Read the model definition and answer for the solid it produces. Units are mm, in the model's axes. A direction names the side the tool comes from. Give positions to 0.01 mm unless a question says otherwise; leave off trailing zeros. Order: outer loops, then holes, each group sorted by start corner. A loop starts at its lowest first (then second) coordinate and runs counter-clockwise, first axis right, second up. Notation, with made-up numbers: M 75.5,42.25 L 100.5,42.25 A22 ccw 100.5,55.25 Z; hole C 63.25,75 d8. An arc over 180 degrees is marked long. Write item = value, one per line. Start each with the question number.
from build123d import *

# Parameters (mm, degrees)
BOSS_EXTRUDE1_DEPTH = 1168.4
CUT_EXTRUDE1_REACH  = 27.4
SKETCH2_R           = 2.667
CUT_EXTRUDE2_REACH  = 27.4
SKETCH3_R           = 2.5527


with BuildPart() as part:
    # Sketch1 → Boss-Extrude1 (new body)
    with BuildSketch(Plane(origin=(0, 0, 0), x_dir=(1, 0, 0), z_dir=(0, 1, 0))):
        Polygon((3.175, 3.175), (3.175, 25.4), (0, 25.4), (0, 0), (50.8, 0), (50.8, 25.4), (47.625, 25.4), (47.625, 3.175), align=None)
    extrude(amount=BOSS_EXTRUDE1_DEPTH)

    # Sketch2 → Cut-Extrude1 (cut, up to next)
    with BuildSketch(Plane.XY, mode=Mode.PRIVATE) as cut_extrude1_sk1:
        with Locations((25.4, 76.2)):
            Circle(SKETCH2_R)
    cut_extrude1_tool1 = extrude(cut_extrude1_sk1.sketch, amount=-CUT_EXTRUDE1_REACH, mode=Mode.PRIVATE) & part.part
    add(cut_extrude1_tool1.solids().sort_by_distance((25.4, 76.2, 0))[0], mode=Mode.SUBTRACT)
    # Sketch2 → Cut-Extrude1 (cut, up to next)
    with BuildSketch(Plane.XY, mode=Mode.PRIVATE) as cut_extrude1_sk2:
        with Locations((25.4, 136.144)):
            Circle(SKETCH2_R)
    cut_extrude1_tool2 = extrude(cut_extrude1_sk2.sketch, amount=-CUT_EXTRUDE1_REACH, mode=Mode.PRIVATE) & part.part
    add(cut_extrude1_tool2.solids().sort_by_distance((25.4, 136.144, 0))[0], mode=Mode.SUBTRACT)
    # Sketch2 → Cut-Extrude1 (cut, up to next)
    with BuildSketch(Plane.XY, mode=Mode.PRIVATE) as cut_extrude1_sk3:
        with Locations((25.4, 196.088)):
            Circle(SKETCH2_R)
    cut_extrude1_tool3 = extrude(cut_extrude1_sk3.sketch, amount=-CUT_EXTRUDE1_REACH, mode=Mode.PRIVATE) & part.part
    add(cut_extrude1_tool3.solids().sort_by_distance((25.4, 196.088, 0))[0], mode=Mode.SUBTRACT)
    # Sketch2 → Cut-Extrude1 (cut, up to next)
    with BuildSketch(Plane.XY, mode=Mode.PRIVATE) as cut_extrude1_sk4:
        with Locations((25.4, 256.032)):
            Circle(SKETCH2_R)
    cut_extrude1_tool4 = extrude(cut_extrude1_sk4.sketch, amount=-CUT_EXTRUDE1_REACH, mode=Mode.PRIVATE) & part.part
    add(cut_extrude1_tool4.solids().sort_by_distance((25.4, 256.032, 0))[0], mode=Mode.SUBTRACT)
    # Sketch2 → Cut-Extrude1 (cut, up to next)
    with BuildSketch(Plane.XY, mode=Mode.PRIVATE) as cut_extrude1_sk5:
        with Locations((25.4, 315.976)):
            Circle(SKETCH2_R)
    cut_extrude1_tool5 = extrude(cut_extrude1_sk5.sketch, amount=-CUT_EXTRUDE1_REACH, mode=Mode.PRIVATE) & part.part
    add(cut_extrude1_tool5.solids().sort_by_distance((25.4, 315.976, 0))[0], mode=Mode.SUBTRACT)
    # Sketch2 → Cut-Extrude1 (cut, up to next)
    with BuildSketch(Plane.XY, mode=Mode.PRIVATE) as cut_extrude1_sk6:
        with Locations((25.4, 375.92)):
            Circle(SKETCH2_R)
    cut_extrude1_tool6 = extrude(cut_extrude1_sk6.sketch, amount=-CUT_EXTRUDE1_REACH, mode=Mode.PRIVATE) & part.part
    add(cut_extrude1_tool6.solids().sort_by_distance((25.4, 375.92, 0))[0], mode=Mode.SUBTRACT)
    # Sketch2 → Cut-Extrude1 (cut, up to next)
    with BuildSketch(Plane.XY, mode=Mode.PRIVATE) as cut_extrude1_sk7:
        with Locations((25.4, 435.864)):
            Circle(SKETCH2_R)
    cut_extrude1_tool7 = extrude(cut_extrude1_sk7.sketch, amount=-CUT_EXTRUDE1_REACH, mode=Mode.PRIVATE) & part.part
    add(cut_extrude1_tool7.solids().sort_by_distance((25.4, 435.864, 0))[0], mode=Mode.SUBTRACT)
    # Sketch2 → Cut-Extrude1 (cut, up to next)
    with BuildSketch(Plane.XY, mode=Mode.PRIVATE) as cut_extrude1_sk8:
        with Locations((25.4, 495.808)):
            Circle(SKETCH2_R)
    cut_extrude1_tool8 = extrude(cut_extrude1_sk8.sketch, amount=-CUT_EXTRUDE1_REACH, mode=Mode.PRIVATE) & part.part
    add(cut_extrude1_tool8.solids().sort_by_distance((25.4, 495.808, 0))[0], mode=Mode.SUBTRACT)
    # Sketch2 → Cut-Extrude1 (cut, up to next)
    with BuildSketch(Plane.XY, mode=Mode.PRIVATE) as cut_extrude1_sk9:
        with Locations((25.4, 555.752)):
            Circle(SKETCH2_R)
    cut_extrude1_tool9 = extrude(cut_extrude1_sk9.sketch, amount=-CUT_EXTRUDE1_REACH, mode=Mode.PRIVATE) & part.part
    add(cut_extrude1_tool9.solids().sort_by_distance((25.4, 555.752, 0))[0], mode=Mode.SUBTRACT)
    # Sketch2 → Cut-Extrude1 (cut, up to next)
    with BuildSketch(Plane.XY, mode=Mode.PRIVATE) as cut_extrude1_sk10:
        with Locations((25.4, 615.696)):
            Circle(SKETCH2_R)
    cut_extrude1_tool10 = extrude(cut_extrude1_sk10.sketch, amount=-CUT_EXTRUDE1_REACH, mode=Mode.PRIVATE) & part.part
    add(cut_extrude1_tool10.solids().sort_by_distance((25.4, 615.696, 0))[0], mode=Mode.SUBTRACT)
    # Sketch2 → Cut-Extrude1 (cut, up to next)
    with BuildSketch(Plane.XY, mode=Mode.PRIVATE) as cut_extrude1_sk11:
        with Locations((25.4, 675.64)):
            Circle(SKETCH2_R)
    cut_extrude1_tool11 = extrude(cut_extrude1_sk11.sketch, amount=-CUT_EXTRUDE1_REACH, mode=Mode.PRIVATE) & part.part
    add(cut_extrude1_tool11.solids().sort_by_distance((25.4, 675.64, 0))[0], mode=Mode.SUBTRACT)
    # Sketch2 → Cut-Extrude1 (cut, up to next)
    with BuildSketch(Plane.XY, mode=Mode.PRIVATE) as cut_extrude1_sk12:
        with Locations((25.4, 735.584)):
            Circle(SKETCH2_R)
    cut_extrude1_tool12 = extrude(cut_extrude1_sk12.sketch, amount=-CUT_EXTRUDE1_REACH, mode=Mode.PRIVATE) & part.part
    add(cut_extrude1_tool12.solids().sort_by_distance((25.4, 735.584, 0))[0], mode=Mode.SUBTRACT)
    # Sketch2 → Cut-Extrude1 (cut, up to next)
    with BuildSketch(Plane.XY, mode=Mode.PRIVATE) as cut_extrude1_sk13:
        with Locations((25.4, 795.528)):
            Circle(SKETCH2_R)
    cut_extrude1_tool13 = extrude(cut_extrude1_sk13.sketch, amount=-CUT_EXTRUDE1_REACH, mode=Mode.PRIVATE) & part.part
    add(cut_extrude1_tool13.solids().sort_by_distance((25.4, 795.528, 0))[0], mode=Mode.SUBTRACT)
    # Sketch2 → Cut-Extrude1 (cut, up to next)
    with BuildSketch(Plane.XY, mode=Mode.PRIVATE) as cut_extrude1_sk14:
        with Locations((25.4, 855.472)):
            Circle(SKETCH2_R)
    cut_extrude1_tool14 = extrude(cut_extrude1_sk14.sketch, amount=-CUT_EXTRUDE1_REACH, mode=Mode.PRIVATE) & part.part
    add(cut_extrude1_tool14.solids().sort_by_distance((25.4, 855.472, 0))[0], mode=Mode.SUBTRACT)
    # Sketch2 → Cut-Extrude1 (cut, up to next)
    with BuildSketch(Plane.XY, mode=Mode.PRIVATE) as cut_extrude1_sk15:
        with Locations((25.4, 915.416)):
            Circle(SKETCH2_R)
    cut_extrude1_tool15 = extrude(cut_extrude1_sk15.sketch, amount=-CUT_EXTRUDE1_REACH, mode=Mode.PRIVATE) & part.part
    add(cut_extrude1_tool15.solids().sort_by_distance((25.4, 915.416, 0))[0], mode=Mode.SUBTRACT)
    # Sketch2 → Cut-Extrude1 (cut, up to next)
    with BuildSketch(Plane.XY, mode=Mode.PRIVATE) as cut_extrude1_sk16:
        with Locations((25.4, 975.36)):
            Circle(SKETCH2_R)
    cut_extrude1_tool16 = extrude(cut_extrude1_sk16.sketch, amount=-CUT_EXTRUDE1_REACH, mode=Mode.PRIVATE) & part.part
    add(cut_extrude1_tool16.solids().sort_by_distance((25.4, 975.36, 0))[0], mode=Mode.SUBTRACT)
    # Sketch2 → Cut-Extrude1 (cut, up to next)
    with BuildSketch(Plane.XY, mode=Mode.PRIVATE) as cut_extrude1_sk17:
        with Locations((25.4, 1035.304)):
            Circle(SKETCH2_R)
    cut_extrude1_tool17 = extrude(cut_extrude1_sk17.sketch, amount=-CUT_EXTRUDE1_REACH, mode=Mode.PRIVATE) & part.part
    add(cut_extrude1_tool17.solids().sort_by_distance((25.4, 1035.304, 0))[0], mode=Mode.SUBTRACT)
    # Sketch2 → Cut-Extrude1 (cut, up to next)
    with BuildSketch(Plane.XY, mode=Mode.PRIVATE) as cut_extrude1_sk18:
        with Locations((25.4, 1095.248)):
            Circle(SKETCH2_R)
    cut_extrude1_tool18 = extrude(cut_extrude1_sk18.sketch, amount=-CUT_EXTRUDE1_REACH, mode=Mode.PRIVATE) & part.part
    add(cut_extrude1_tool18.solids().sort_by_distance((25.4, 1095.248, 0))[0], mode=Mode.SUBTRACT)

    # Sketch3 → Cut-Extrude2 (cut, up to next)
    with BuildSketch(Plane.XY, mode=Mode.PRIVATE) as cut_extrude2_sk1:
        with Locations((25.4, 32.131)):
            Circle(SKETCH3_R)
    cut_extrude2_tool1 = extrude(cut_extrude2_sk1.sketch, amount=-CUT_EXTRUDE2_REACH, mode=Mode.PRIVATE) & part.part
    add(cut_extrude2_tool1.solids().sort_by_distance((25.4, 32.131, 0))[0], mode=Mode.SUBTRACT)
    # Sketch3 → Cut-Extrude2 (cut, up to next)
    with BuildSketch(Plane.XY, mode=Mode.PRIVATE) as cut_extrude2_sk2:
        with Locations((25.4, 14.2875)):
            Circle(SKETCH3_R)
    cut_extrude2_tool2 = extrude(cut_extrude2_sk2.sketch, amount=-CUT_EXTRUDE2_REACH, mode=Mode.PRIVATE) & part.part
    add(cut_extrude2_tool2.solids().sort_by_distance((25.4, 14.2875, 0))[0], mode=Mode.SUBTRACT)


solid = part.part
1) Find the intervals of material crossed by probe 1 along X at (y, z) = (1019, -17.5) (3 decimals); probe 2 along Z at (x, y) = (19.5, 279.5) (3 decimals), in increasing order. Write a range as [from, to].
2) Find section A-A on z = -13. Determine the outline of the cut face in (x, y) (3 decimals).
3) For faces 1 (the face through (27, 0, -2)), 2 (the face through (3.175, 576, -14)), determine the directions among +Z, -Z, +X, -X, +Y, -Y from which every point of the face is accessible in a straight line to the end or side of a thin tool.
4) Find section B-B on y = 180.5. Determine the outline of the cut face in (x, z) (3 decimals).
5) For a pull along X with two mould halves and no side action, classify faces 3 (the face through (50.8, 576, -13)), 4 (the face through (26, 576, -3.175)), 5 (the face through (0, 576, -13)) as pulls with the +X half, pulls with the -X half, needs draft (parallel to the pull), parting line crosses it, or undercut.
6) This flat-tipped pin is pushed along its axis until it touches: P1, Ø8.5, axis at x = 25.4, y = 615.696, coming from the -Z side (3 decimals). Where does it stop, or does it pass through?
Numbers:
q1.probe_1 = [0, 3.175], [47.625, 50.8]
q1.probe_2 = [-3.175, 0]
q2.outline = M 0,0 L 3.175,0 L 3.175,1168.4 L 0,1168.4 Z; M 47.625,0 L 50.8,0 L 50.8,1168.4 L 47.625,1168.4 Z
q3.face_1 = +Z, -Z, +X, -X, -Y
q3.face_2 = -Z, +Y, -Y
q4.outline = M 0,-25.4 L 3.175,-25.4 L 3.175,-3.175 L 47.625,-3.175 L 47.625,-25.4 L 50.8,-25.4 L 50.8,0 L 0,0 Z
q5.face_3 = pulls with the +X half
q5.face_4 = undercut
q5.face_5 = pulls with the -X half
q6.P1 = -3.175
